Geometry: final body of the model. Coordinates: model frame, mm. Face numbers are marked on the shaded views. A direction names the side the tool comes from. Give positions to 0.01 mm unless a question says otherwise; leave off trailing zeros. Write each loop counter-clockwise with the first axis right and the second up, starting at its lowest first coordinate (ties: lowest second). Pieces come first, ordered by that corner, then holes.
Q1. Line query: line 1 (Y direction, x = -5.5, z = 6); line 2 (Y direction, x = 47.5, z = 1.25); line 3 (X direction, y = 13, z = 5). Output: solid intervals per line, ascending.
Q2. Section D-D (x = 5). Return the cut outline in (y, z), plus the area to 3 significant figures.
Q3. Section B-B (y = -7). Return the cut outline in (x, z), plus the area to 3 significant figures.
Q4. Reachability of the marked faces 4, 5, 6, 7 and 8 from +Z, -Z, +X, -X, +Y, -Y: full face, straight path, thin tool, end or side. Return the list, or none.
Q5. Pin query (flat end, axial travel): pin 1 Ø2 at (y, z) = (-0.5, 6.5) entering from -X; pin 2 Ø2.5 at (y, z) = (12, 5) entering from -X; pin 3 Ø1 at (x, z) = (3, 7) entering from +Y; pin 4 Ø1 at (x, z) = (11, 5.5) entering from -Y. Return the tip coordinate at first contact, or that it passes through.
Q6. Section A-A (x = 42). Return the cut outline in (y, z), plus the area to 3 significant figures.
Q7. Section C-C (z = 3.25). Return the cut outline in (x, y).
Q8. Mould query, pull axis X, two halves, no side actions, for the marked faces 1, 2 and 3. Classes: +X half, -X half, draft (parallel to the pull), parting line (faces both ways), or undercut.
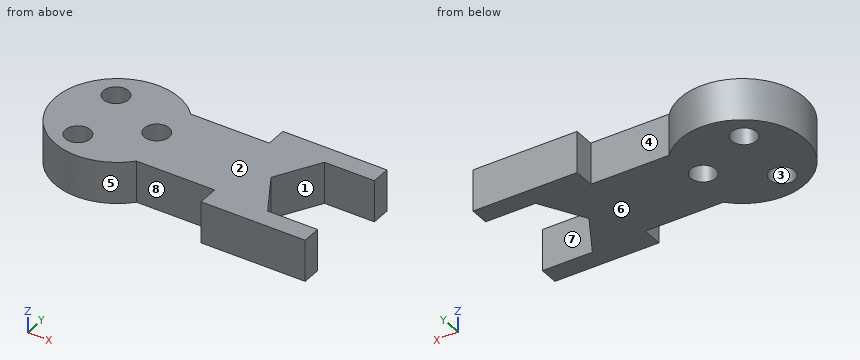
Autodesk Inventor part; units mm, degrees
ref_plane "YZ Plane" through (0, 0, 0) normal (1, 0, 0) x (0, 1, 0)
ref_plane "XZ Plane" through (0, 0, 0) normal (0, 1, 0) x (-1, 0, 0)
ref_plane "XY Plane" through (0, 0, 0) normal (0, 0, 1) x (1, 0, 0)
sketch "Эскиз1" plane through (0, 0, 0) normal (0, 0, 1) x (1, 0, 0)
  point P0 (0, 0)
sketch "Эскиз2" plane through (0, 0, 0) normal (0, 0, 1) x (1, 0, 0)
  circle A0 centre (0, 0) radius 9
  circle A1 centre (0, 0) radius 14.9355
  line L0 (29.9138, -9.957) -> (11.1323, -9.957)
  line L1 (11.0941, 9.9995) -> (29.9138, 9.9995)
  line L2 (11.0941, 9.9995) -> (29.9138, 9.9995)
  line L3 (29.9138, 9.9995) -> (29.9138, 14.9995)
  line L4 (29.9138, 14.9995) -> (54.9138, 14.9995)
  line L5 (29.9138, -9.957) -> (29.9138, -14.9572)
  line L6 (29.9138, -14.9572) -> (54.9138, -14.9572)
  line L7 (-18.0074, -0.0005) -> (54.9138, -0.0005)
  line L8 (54.9138, 14.9995) -> (48.9138, 14.9995)
  line L9 (48.9138, 14.9995) -> (48.9138, -8.0243)
  line L10 (42.9138, 10.3918) -> (54.9138, 10.3918)
  line L11 (54.9138, -10.3928) -> (42.9138, -10.3928)
  line L12 (42.9138, -10.3928) -> (36.9138, -0.0005)
  line L13 (36.9138, -0.0005) -> (42.9138, 10.3918)
  line L14 (54.9138, 14.9995) -> (54.9138, 10.3918)
  line L15 (54.9138, -14.9572) -> (54.9138, -10.3928)
  line L16 (0, 0) -> (22.1205, 0) construction
  line L17 (0, 0) -> (18.5985, 0) construction
  line L18 (0, 0) -> (18.6696, 0) construction
  line L19 (0, 0) -> (12.4111, 0) construction
  circle A2 centre (-5.1622, 7.3724) radius 3
  circle A3 centre (-3.9303, -8.4286) radius 3
  circle A4 centre (8.9658, 0.7844) radius 3
  point P0 (48.9138, -0.0005)
  point P1 (48.9138, -0.0005)
  point P2 (48.9138, -0.0005)
extrude "Выдавливание1" add sketch "Эскиз2" along normal blind 10 contours A4 L7 A0 A2 | A0 A2 L7 A1 A4 | A4 L7 A1 A0 A3 | A0 A3 L7 A4 | L7 L12 L11 L15 L6 L5 L0 A1 | A1 L1 L3 L4 L9 L10 L13 L7 | L9 L4 L14 L10
Computed:
1. line 1: y = -13.89 to -10.99, -5.87 to 4.39, 10.35 to 13.89
1. line 2: y = -14.96 to -10.39, 10.39 to 15
1. line 3: x = -7.35 to 7.35, 29.91 to 54.91
2. outline: (-14.07, 0) - (14.07, 0) - (14.07, 10) - (-14.07, 10) - close
2. area: 281 mm2
3. outline: (-13.19, 0) - (-6.57, 0) - (-6.57, 10) - (-13.19, 10) - close; (-1.29, 0) - (40.95, 0) - (40.95, 10) - (-1.29, 10) - close
3. area: 489 mm2
4. face 4: +Z, -Z, +Y
4. face 5: +Z, -Z
4. face 6: -Z, +X, -X, +Y, -Y
4. face 7: +Z, -Z, +X
4. face 8: +Z, -Z, -Y
5. pin 1: stops at x = -14.94
5. pin 2: stops at x = -10.37
5. pin 3: stops at y = 14.72
5. pin 4: stops at y = -10.62
6. outline: (-14.96, 0) - (-8.81, 0) - (-8.81, 10) - (-14.96, 10) - close; (8.81, 0) - (15, 0) - (15, 10) - (8.81, 10) - close
6. area: 123 mm2
7. outline: (11.09, 10) arc R14.94 ccw (long way) to (11.13, -9.96) - (29.91, -9.96) - (29.91, -14.96) - (54.91, -14.96) - (54.91, -10.39) - (42.91, -10.39) - (36.91, 0) - (42.91, 10.39) - (54.91, 10.39) - (54.91, 15) - (29.91, 15) - (29.91, 10) - close; hole circle Ø6 at (-5.16, 7.37); hole circle Ø6 at (-3.93, -8.43); hole circle Ø6 at (8.97, 0.78)
8. face 1: +X half
8. face 2: draft
8. face 3: undercut
